Can you work these out from the drawing? Everything is in mm from the part's minimum corner. A direction names the side the tool comes from. Coordinates: 2 decimals unless noted, no trailing zeros. Loops run counter-clockwise (first coordinate to the right, second up) from the corner with the lowest first, then second, coordinate; pieces in that order, holes last. Notation, with made-up numbers: M -10,30.5 L 9,30.5 A24 ccw 9,51.5 Z; hole C 20,59.5 d10. An arc over 180 degrees is marked long. Use CSV: the item, a comma, the result in double quotes. Start each with the question number.
Q1. If we mould it in two halves opening along Y, with no side actions, what happens to the marked faces 1, 2 and 3? For each: +Y half, -Y half, draft (parallel to the pull), parting line (faces both ways), or undercut.
Q2. Which directions (+Z, -Z, +X, -X, +Y, -Y) give clear straight access to the entire face, cutting with the end or side of a thin tool? Please do the marked faces 4 and 5.
Q3. Please list where these lines run through material, in increasing order: probe 1 along Z at (x, y) = (12.5, 5.5); probe 2 along Y at (x, z) = (17.75, 2.5); probe 3 along X at (y, z) = (2.75, 13.75). Write a range as [from, to].
Q4. If we section it at D-D (y = 11.25): Please give me the cut outline in (x, z).
Q5. If we section it at C-C (x = 3.5): Please give me the cut outline in (y, z), and give its area (3 significant figures).
Q6. If we section it at A-A (y = 6.35): Please give me the cut outline in (x, z).
Q7. If we section it at B-B (z = 23.5): Please give me the cut outline in (x, y), and give its area (3 significant figures).
Q8. For pin 1 Ø4 at (x, y) = (7, 5) entering from -Z; pin 2 Ø1 at (x, z) = (22.5, 17.5) entering from +Y; pin 3 Ø2 at (x, z) = (9.5, 8.5) entering from -Y, each with a flat end and sliding along its axis, tell me the tip position at first contact or that it passes through.
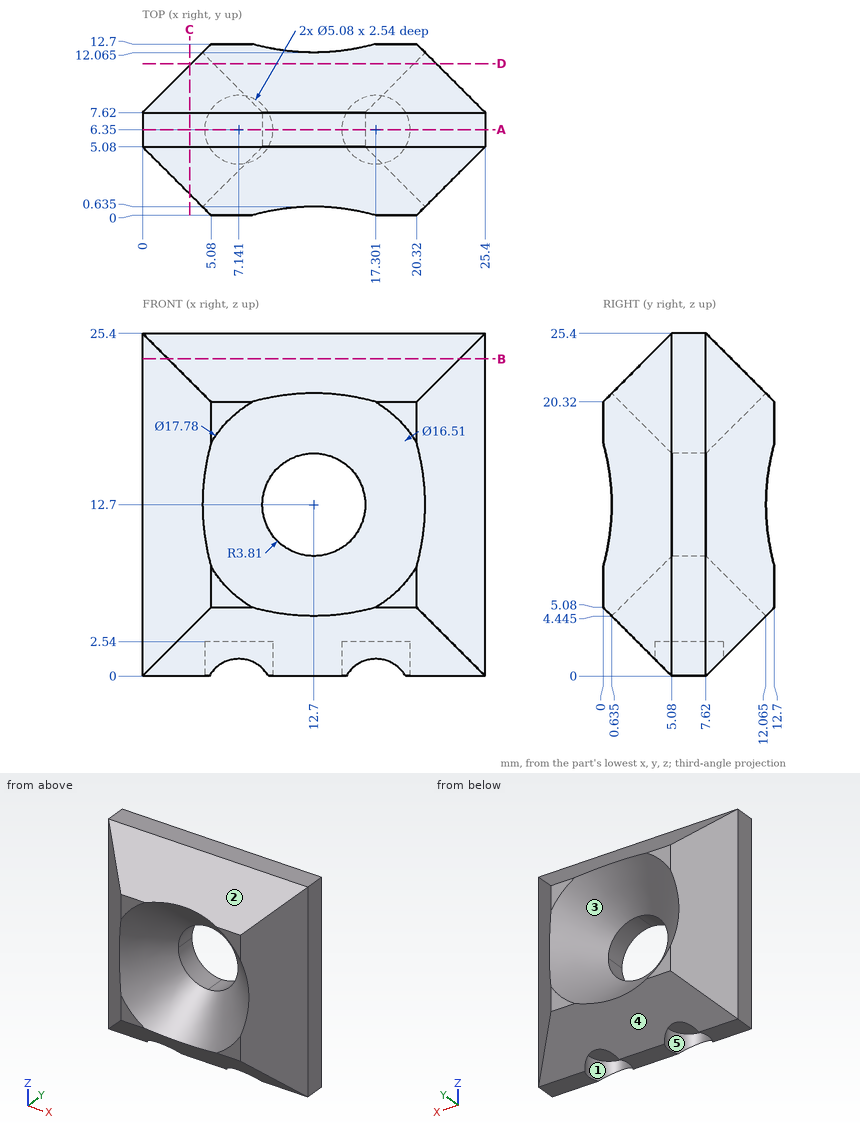
Results below:
1,face 1,"undercut"
1,face 2,"-Y half"
1,face 3,"+Y half"
2,face 4,"-Z, +X, -X, +Y"
2,face 5,"-Z"
3,probe 1,"[0, 8.9], [16.5, 25.4]"
3,probe 2,"[2.58, 3.85], [8.85, 10.12]"
3,probe 3,"[2.33, 6.65], [18.75, 23.07]"
4,outline,"M 3.63,3.63 L 21.77,3.63 L 21.77,21.77 L 3.63,21.77 Z; hole C 12.7,12.7 d14.88"
5,outline,"M 1.58,3.5 L 5.08,0 L 7.62,0 L 11.12,3.5 L 11.12,21.9 L 7.62,25.4 L 5.08,25.4 L 1.58,21.9 Z"
5,area,"218 mm^2"
6,outline,"M 0,0 L 4.6,0 L 4.6,2.54 L 9.68,2.54 L 9.68,0 L 14.76,0 L 14.76,2.54 L 19.84,2.54 L 19.84,0 L 25.4,0 L 25.4,25.4 L 0,25.4 Z; hole C 12.7,12.7 d7.62"
7,outline,"M 0,5.08 L 1.9,3.18 L 23.5,3.18 L 25.4,5.08 L 25.4,7.62 L 23.5,9.52 L 1.9,9.52 L 0,7.62 Z"
7,area,"154 mm^2"
8,pin 1,"z = 0.1"
8,pin 2,"y = 11.02"
8,pin 3,"y = 2.61"
